```python
from build123d import *

# Parameters (mm, degrees)
SKETCH1_W           = 130
SKETCH1_H           = 20
SKETCH1_R           = 1.5
BOSS_EXTRUDE1_DEPTH = 1
BOSS_EXTRUDE2_START = 26
SKETCH3_R           = 1
SKETCH3_R_2         = 0.5
BOSS_EXTRUDE2_DEPTH = 26
LPATTERN1_COUNT     = 2
LPATTERN1_PITCH     = 52


with BuildPart() as part:
    # Sketch1 → Boss-Extrude1 (new body)
    with BuildSketch(Plane.XY):
        with Locations((65, 10)):
            Rectangle(SKETCH1_W, SKETCH1_H)
        with Locations((65, 10.5)):
            Circle(SKETCH1_R, mode=Mode.SUBTRACT)
        with Locations((5, 10.5)):
            Circle(SKETCH1_R, mode=Mode.SUBTRACT)
        with Locations((125, 10.5)):
            Circle(SKETCH1_R, mode=Mode.SUBTRACT)
    extrude(amount=BOSS_EXTRUDE1_DEPTH)

    # Sketch3 → Boss-Extrude2 (add)
    with BuildSketch(Plane(origin=(0, 0, 0), x_dir=(0, 0, -1), z_dir=(1, 0, 0)).offset(BOSS_EXTRUDE2_START)):
        with Locations((-0.863530112, 20.504297279)):
            Circle(SKETCH3_R)
        with Locations((-0.863530112, 20.504297279)):
            Circle(SKETCH3_R_2, mode=Mode.SUBTRACT)
    boss_extrude2 = extrude(amount=BOSS_EXTRUDE2_DEPTH)

    # LPattern1: Boss-Extrude2 ×2
    with Locations(*[(i * LPATTERN1_PITCH, 0, 0) for i in range(1, LPATTERN1_COUNT)]):
        add(boss_extrude2)


solid = part.part
```
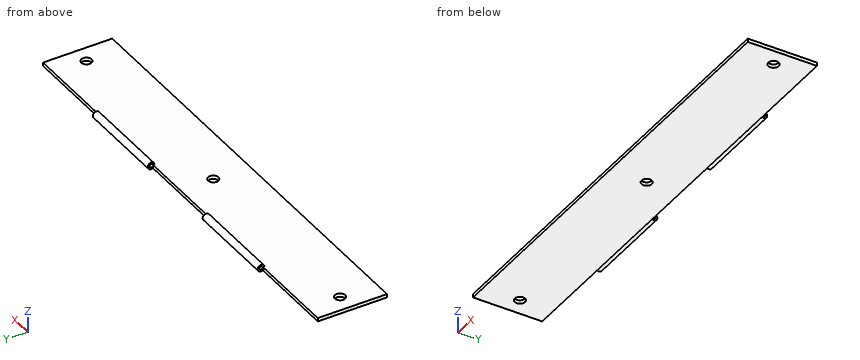
Here's how the part is built. I have some questions about the finished solid (model axes, mm). Give positions to 0.01 mm unless a question says otherwise; leave off trailing zeros. Loops run counter-clockwise (first coordinate to the right, second up) from the corner with the lowest first, then second, coordinate; pieces in that order, holes last. Notation, with made-up numbers: M 30.25,-2.5 L 50.25,-2.5 A15 cw 50.25,5.5 Z; hole C 14,78.5 d10. An arc over 180 degrees is marked long. Return JSON: item names as keys, results as strings.
Item 1: Imagine slicing it at C-C on x = 36.5. List the corners of the cut face in (y, z) for me, then the cut area to 3 significant figures.
A:
{"outline": "M 0,0 L 20,0 A1 ccw long 19.51,1 L 0,1 Z; hole C 20.5,0.86 d1", "area": "22.0 mm^2"}
Item 2: I'm going to push flat-ended pins straight in: pin 1 Ø3.5 at (x, y) = (5, 10.5) entering from -Z; pin 2 Ø10 at (x, y) = (42.5, 13) entering from +Z; pin 3 Ø2.5 at (x, y) = (125, 10.5) entering from +Z; pin 4 Ø1.1 at (x, z) = (15, 0.5) entering from +Y. Where does each tip first touch, or does it pass through?
A:
{"pin 1": "stops at z = 0", "pin 2": "stops at z = 1", "pin 3": "passes through", "pin 4": "stops at y = 20"}
Item 3: Imagine slicing it at D-D on x = 118.5. List the corners of the cut face in (y, z) for me, then the cut area to 3 significant figures.
A:
{"outline": "M 0,0 L 20,0 L 20,1 L 0,1 Z", "area": "20.0 mm^2"}
Item 4: Imagine slicing it at B-B on x = 5. List the corners of the cut face in (y, z) for me.
A:
{"outline": "M 0,0 L 9,0 L 9,1 L 0,1 Z; M 12,0 L 20,0 L 20,1 L 12,1 Z"}
Item 5: Imagine slicing it at A-A on y = 10.5. List the corners of the cut face in (x, z) for me, then the cut area to 3 significant figures.
A:
{"outline": "M 0,0 L 3.5,0 L 3.5,1 L 0,1 Z; M 6.5,0 L 63.5,0 L 63.5,1 L 6.5,1 Z; M 66.5,0 L 123.5,0 L 123.5,1 L 66.5,1 Z; M 126.5,0 L 130,0 L 130,1 L 126.5,1 Z", "area": "121 mm^2"}
Item 6: Please list where these lines run through material, in increasing order: line 1 (Y direction, x = 65, z = 0.55); line 2 (Y direction, x = 7, z = 0.6); line 3 (Z direction, x = 55.5, y = 13.5).
A:
{"line 1": "y = 0 to 9, 12 to 20", "line 2": "y = 0 to 20", "line 3": "z = 0 to 1"}
